Autodesk Inventor part; units mm, degrees
ref_plane "YZ Plane" through (0, 0, 0) normal (1, 0, 0) x (0, 1, 0)
ref_plane "XZ Plane" through (0, 0, 0) normal (0, 1, 0) x (-1, 0, 0)
ref_plane "XY Plane" through (0, 0, 0) normal (0, 0, 1) x (1, 0, 0)
sketch "スケッチ1" plane through (0, 0, 0) normal (0, 0, 1) x (1, 0, 0)
  line L0 (-72.5, -21.65) -> (72.5, -21.65) construction
  line L1 (72.5, -21.65) -> (72.5, 21.65) construction
  line L2 (72.5, 21.65) -> (-72.5, 21.65) construction
  line L3 (-72.5, 21.65) -> (-72.5, -21.65) construction
  line L4 (-72.5, -21.65) -> (72.5, 21.65) construction
  line L5 (72.5, -21.65) -> (-72.5, 21.65) construction
  line L6 (-67.5, 21.65) -> (-67.5, -21.65) construction
  line L7 (0, 0) -> (0, 21.65) construction
  line L8 (0, 0) -> (-72.5, 0) construction
  line L9 (67.5, 21.65) -> (67.5, -21.65) construction
  line L10 (-72.5, -21.65) -> (-61.6, -21.65)
  line L11 (49.5, 21.65) -> (49.5, 23.65)
  line L12 (49.5, 23.65) -> (62.5, 23.65)
  line L13 (62.5, 23.65) -> (62.5, 21.65)
  line L14 (66.6, 21.65) -> (72.5, 21.65)
  line L15 (72.5, 21.65) -> (72.5, -21.65)
  line L16 (72.5, -21.65) -> (61.6, -21.65)
  line L17 (-57.5, -21.65) -> (-57.5, -23.65)
  line L18 (-57.5, -23.65) -> (57.5, -23.65)
  line L19 (57.5, -23.65) -> (57.5, -21.65)
  arc A0 (45.4, 21.65) -> (49.5, 21.65) centre (47.45, 21.65) ccw
  arc A1 (62.5, 21.65) -> (66.6, 21.65) centre (64.55, 21.65) ccw
  arc A2 (-57.5, -21.65) -> (-61.6, -21.65) centre (-59.55, -21.65) ccw
  arc A3 (61.6, -21.65) -> (57.5, -21.65) centre (59.55, -21.65) ccw
  line L20 (-72.5, -21.65) -> (-72.5, -16.65)
  line L21 (-72.5, -16.65) -> (39.5, 21.65)
  line L22 (45.4, 21.65) -> (39.5, 21.65)
  line L23 (66.95, 24.476) -> (70.05, 24.476) construction
  line L24 (70.05, 24.476) -> (70.05, 13.3235) construction
  line L25 (70.05, 13.3235) -> (66.95, 13.3235) construction
  line L26 (66.95, 13.3235) -> (66.95, 24.476) construction
  line L27 (68.5, 24.476) -> (68.5, 13.3235) construction
  line L28 (41.95, 24.476) -> (45.05, 24.476) construction
  line L29 (45.05, 24.476) -> (45.05, 13.9945) construction
  line L30 (45.05, 13.9945) -> (41.95, 13.9945) construction
  line L31 (41.95, 13.9945) -> (41.95, 24.476) construction
  line L32 (43.5, 24.476) -> (43.5, 13.9945) construction
  dimension "d16" = 5
  dimension "d20" = 43.3
  dimension "d40" = 135
  dimension "d41" = 10
  dimension "d42" = 2.05
  dimension "d43" = 2
  dimension "d44" = 5
  dimension "d45" = 10
  dimension "d46" = 10
  dimension "d48" = 3.1
  dimension "d50" = 4
  dimension "d51" = 25
  dimension "d52" = 3.1
  dimension "d62" = 6
  dimension "d63" = 6
extrude "押し出し1" add sketch "スケッチ1" along normal blind 2.5
mirror "ミラー1" about plane through (8.3734, -6.8299, 0) normal (0, 0, -1) of "押し出し1"
sketch "スケッチ2" plane through (-72.5, -21.65, 2.5) normal (0, -1, 0) x (1, 0, 0)
  line L0 (0, -5) -> (0, 0)
  line L1 (15, -5) -> (130, -5) construction
  line L2 (72.5, -5) -> (72.5, 0) construction
  line L3 (15, 0) -> (130, 0) construction
  point P0 (72.5, -2.5)
  point P1 (140, -2.5)
  point P2 (0, -2.5)
hole "穴1" at (67.5, -21.65, 0) direction (0, 1, 0) diameter 2.459 depth 2
sketch "スケッチ4" plane through (66.6, 21.65, 2.5) normal (0, 1, 0) x (1, 0, 0)
  line L0 (5.9, 5) -> (5.9, 0)
  point P0 (-66.6, 2.5)
  point P1 (1.9, 2.5)
  point P2 (-23.1, 2.5)
  point P3 (5.9, 2.5)
  dimension "d53" = 4
  dimension "d54" = 25
hole "穴2" at (68.5, 21.65, 0) at (43.5, 21.65, 0) direction (0, -1, 0) diameter 2.459 depth 2.5
sketch "スケッチ6" plane through (0, 0, 2.5) normal (0, 0, 1) x (1, 0, 0)
  line L0 (61.6, -21.65) -> (72.5, -21.65)
  line L1 (72.5, -21.65) -> (72.5, 21.65)
  line L2 (72.5, 21.65) -> (66.6, 21.65)
  line L3 (39.5, 21.65) -> (-72.5, -16.65)
  line L4 (67.5, 16.65) -> (67.5, -16.65) construction
  line L5 (67.5, -16.65) -> (-57.0473, -16.65) construction
  line L6 (-57.0473, -16.65) -> (40.3313, 16.65) construction
  line L7 (40.3313, 16.65) -> (67.5, 16.65) construction
  line L8 (67.5, -16.65) -> (-8.358, 0) construction
  line L9 (67.5, -14.0905) -> (67.5, 16.65)
  line L10 (67.5, 16.65) -> (40.3313, 16.65)
  line L11 (40.3313, 16.65) -> (-3.7993, 1.5589)
  line L12 (-3.7993, 1.5589) -> (67.5, -14.0905)
  line L13 (55.8388, -16.65) -> (-57.0473, -16.65)
  line L14 (-57.0473, -16.65) -> (-12.9167, -1.5589)
  line L15 (-12.9167, -1.5589) -> (55.8388, -16.65)
  point P0 (0, 0)
  dimension "d72" = 5
  dimension "d73" = 5
  dimension "d74" = 5
  dimension "d75" = 5
  dimension "d76" = 5
extrude "押し出し4" cut sketch "スケッチ6" against normal blind 10
fillet "フィレット3" radius 3 7 edges at (-3.7993, 1.5589, 0) (40.3313, 16.65, 0) (67.5, -14.0905, 0) (55.8388, -16.65, 0) (-12.9167, -1.5589, 0) (-57.0473, -16.65, 0) (67.5, 16.65, 0)
sketch "スケッチ7" plane through (-72.5, -21.65, 2.5) normal (0, -1, 0) x (1, 0, 0)
  line L0 (0, 0) -> (0, -5)
  line L1 (15, 0) -> (130, 0)
  line L2 (15, -5) -> (130, -5)
  line L3 (0, -2.5) -> (5, -2.5)
  point P0 (72.5, -2.5)
  dimension "d80" = 5
hole "穴3" at (-67.5, -21.65, 0) direction (0, 1, 0) diameter 3 end through all
equation "\"d16\" = d4"
equation "\"d40\" = d6"
equation "\"d41\" = d3"
equation "\"d46\" = d45"
equation "\"d63\" = d62"
equation "\"d73\" = d72"
equation "\"d74\" = d73"
equation "\"d75\" = d74"
equation "\"d76\" = d74"
properties part number "前腕_サブフレーム_1_1" material "アセタール樹脂、黒"
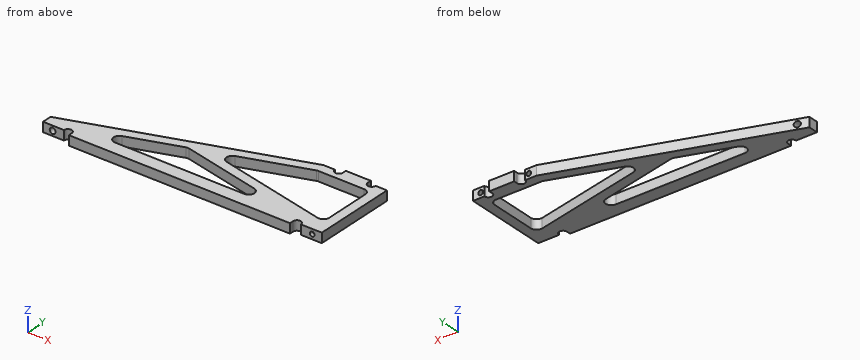
Model file for the job. Use its own axes, mm. Coordinates: 2 decimals unless noted, no trailing zeros. Loops run counter-clockwise (first coordinate to the right, second up) from the corner with the lowest first, then second, coordinate; pieces in that order, holes last. Notation, with made-up numbers: (21.5, 19.25) - (48.5, 19.25) arc R14 ccw to (48.5, 42.25) - close; hole circle Ø11 at (16.5, -5). An arc over 180 degrees is marked (long way). Answer as a JSON object with one key per item and string values. Group by question number.
(1) Cut at B-B (x = 59.55). Give the cut face in (y, z), then the cut area to 3 significant figures.
(2) Cut at D-D (x = -55). Give the cut face in (y, z), then the cut area to 3 significant figures.
(3) Flat gauge pins, fed straight in: pin 1 (2 mm diameter, centred on x = 68.5, z = 0, fed in from +Y); pin 2 (1.5 mm diameter, centred on x = 43, z = -0.5, fed in from +Y); pin 3 (0.6 mm diameter, centred on y = 23, z = -1, fed in from -X). Where does each tip first touch, or does it go through?
(4) Cut at C-C (z = -0.2). State how many separate pieces and enclosed holes the cut face has, then the cut area to 3 significant figures.
(5) Probe line 1 along Y through (x, z) = (64.5, 1.95); line 2 along X through (y, z) = (-21.05, 0); line 3 along X through (y, z) = (-20.3, 0). List the from-to ranges inside material, lowest first.
(6) Cut at A-A (y = 2.5). Give the cut face in (x, z).
Geometry says:
{
 "1": {"outline": "(-19.6, -2.5) - (-12.35, -2.5) - (-12.35, 2.5) - (-19.6, 2.5) - close; (16.65, -2.5) - (23.65, -2.5) - (23.65, 2.5) - (16.65, 2.5) - close", "area": "71.3 mm^2"},
 "2": {"outline": "(-23.65, -2.5) - (-10.67, -2.5) - (-10.67, 2.5) - (-23.65, 2.5) - close", "area": "64.9 mm^2"},
 "3": {"pin 1": "stops at y = 19.15", "pin 2": "stops at y = 21.65", "pin 3": "stops at x = 49.5"},
 "4": {"separate pieces": "2", "enclosed holes": "2", "area": "2,310 mm^2"},
 "5": {"line 1": "y = -21.65 to -13.36, 16.65 to 19.6", "line 2": "x = -72.5 to -69, -66 to -61.51, -57.59 to 57.59, 61.51 to 66.27, 68.73 to 72.5", "line 3": "x = -72.5 to -69, -66 to -61.09, -58.01 to 58.01, 61.09 to 66.27, 68.73 to 72.5"},
 "6": {"outline": "(-16.5, -2.5) - (4.33, -2.5) - (4.33, 2.5) - (-16.5, 2.5) - close; (67.5, -2.5) - (72.5, -2.5) - (72.5, 2.5) - (67.5, 2.5) - close"}
}
